Verification items for the finished model (mm, model axes). Round coordinates to 2 decimals unless told otherwise and drop trailing zeros. Write each loop counter-clockwise with the first axis right and the second up, starting at its lowest first coordinate (ties: lowest second). Pieces come first, ordered by that corner, then holes. Notation, with made-up numbers: M 22,-10 L 79,-10 A10 cw 79,7 Z; hole C 72,-22.75 d10. An arc over 180 degrees is marked long. One line per item, written item: value. Start each with the question number.
Item 1: Gauge pin test, flat end, axial feed: pin 1 (13 mm diameter, centred on x = -20.95, y = 10, fed in from +Z). Record the tip position at first contact, or that the pin passes through.
Item 2: Section check B-B, the plane x = -20.95. Record the cut outline in (y, z).
Item 3: Section check C-C, the plane z = 1.35. Record the cut outline in (x, y).
Item 4: Section check D-D, the plane x = 17. Record the cut outline in (y, z), then the cut area to 3 significant figures.
Item 5: Thickness scan on probe 1 along Y at (x, z) = (20.95, 1.3); probe 2 along X at (y, z) = (14, 4); probe 3 along Y at (x, z) = (-20.5, 1.6). Record the ranges inside material, lowest first. Write a range as from..to.
Item 6: Section check A-A, the plane y = 10. Record the cut outline in (x, z).
from build123d import *

# Parameters (mm, degrees)
SKETCH1_W           = 230
SKETCH1_H           = 90
BOSS_EXTRUDE1_DEPTH = 5
FILLET1_R           = 20
CUT_EXTRUDE1_REACH  = 125.592
SKETCH2_R           = 11
SKETCH2_R_2         = 16.75
CUT_EXTRUDE2_REACH  = 125.592
SKETCH3_R           = 4.65
SKETCH3_R_2         = 4.8


with BuildPart() as part:
    # Sketch1 → Boss-Extrude1 (new body)
    with BuildSketch(Plane.XY):
        Rectangle(SKETCH1_W, SKETCH1_H)
    extrude(amount=BOSS_EXTRUDE1_DEPTH)

    # Fillet1
    fillet1_edges = [part.edges().sort_by_distance(p)[0] for p in [
        (-115, 45, 2.5),
        (115, 45, 2.5),
    ]]
    fillet(fillet1_edges, radius=FILLET1_R)

    # Sketch2 → Cut-Extrude1 (cut, up to next)
    with BuildSketch(Plane.XY.offset(5), mode=Mode.PRIVATE) as cut_extrude1_sk1:
        with Locations((-20.95, 10)):
            Circle(SKETCH2_R)
    cut_extrude1_tool1 = extrude(cut_extrude1_sk1.sketch, amount=-CUT_EXTRUDE1_REACH, mode=Mode.PRIVATE) & part.part
    # Sketch2 → Cut-Extrude1 (cut, up to next)
    with BuildSketch(Plane.XY.offset(5), mode=Mode.PRIVATE) as cut_extrude1_sk2:
        with Locations((20.95, 10)):
            Circle(SKETCH2_R)
    cut_extrude1_tool2 = extrude(cut_extrude1_sk2.sketch, amount=-CUT_EXTRUDE1_REACH, mode=Mode.PRIVATE) & part.part
    # Sketch2 → Cut-Extrude1 (cut, up to next)
    with BuildSketch(Plane.XY.offset(5), mode=Mode.PRIVATE) as cut_extrude1_sk3:
        with Locations((49.976927154, -10)):
            Circle(SKETCH2_R_2)
    cut_extrude1_tool3 = extrude(cut_extrude1_sk3.sketch, amount=-CUT_EXTRUDE1_REACH, mode=Mode.PRIVATE) & part.part
    add(cut_extrude1_tool1.solids().sort_by_distance((-20.95, 10, 5))[0], mode=Mode.SUBTRACT)
    add(cut_extrude1_tool2.solids().sort_by_distance((20.95, 10, 5))[0], mode=Mode.SUBTRACT)
    add(cut_extrude1_tool3.solids().sort_by_distance((49.976927, -10, 5))[0], mode=Mode.SUBTRACT)

    # Sketch3 → Cut-Extrude2 (cut, up to next)
    with BuildSketch(Plane(origin=(0, 0, 0), x_dir=(-1, 0, 0), z_dir=(0, 0, -1)), mode=Mode.PRIVATE) as cut_extrude2_sk1:
        with Locations((-42.861480484, 27.315297382)):
            Circle(SKETCH3_R)
    cut_extrude2_tool1 = extrude(cut_extrude2_sk1.sketch, amount=-CUT_EXTRUDE2_REACH, mode=Mode.PRIVATE) & part.part
    # Sketch3 → Cut-Extrude2 (cut, up to next)
    with BuildSketch(Plane(origin=(0, 0, 0), x_dir=(-1, 0, 0), z_dir=(0, 0, -1)), mode=Mode.PRIVATE) as cut_extrude2_sk2:
        with Locations((-88.015918911, -8.560303387)):
            Circle(SKETCH3_R)
    cut_extrude2_tool2 = extrude(cut_extrude2_sk2.sketch, amount=-CUT_EXTRUDE2_REACH, mode=Mode.PRIVATE) & part.part
    # Sketch3 → Cut-Extrude2 (cut, up to next)
    with BuildSketch(Plane(origin=(0, 0, 0), x_dir=(-1, 0, 0), z_dir=(0, 0, -1)), mode=Mode.PRIVATE) as cut_extrude2_sk3:
        with Locations((-16.935196723, -27.604446885)):
            Circle(SKETCH3_R_2)
    cut_extrude2_tool3 = extrude(cut_extrude2_sk3.sketch, amount=-CUT_EXTRUDE2_REACH, mode=Mode.PRIVATE) & part.part
    add(cut_extrude2_tool1.solids().sort_by_distance((42.86148, 27.315297, 0))[0], mode=Mode.SUBTRACT)
    add(cut_extrude2_tool2.solids().sort_by_distance((88.015919, -8.560303, 0))[0], mode=Mode.SUBTRACT)
    add(cut_extrude2_tool3.solids().sort_by_distance((16.935197, -27.604447, 0))[0], mode=Mode.SUBTRACT)


solid = part.part
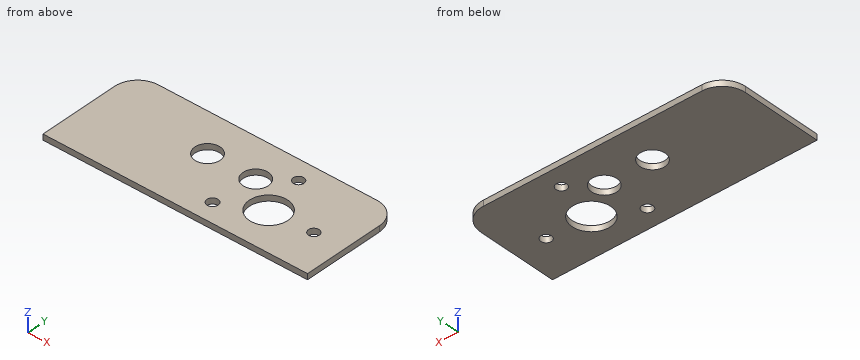
Response values:
1. pin 1: passes through
2. outline: M -45,0 L -1,0 L -1,5 L -45,5 Z; M 21,0 L 45,0 L 45,5 L 21,5 Z
3. outline: M -115,-45 L 115,-45 L 115,25 A20 ccw 95,45 L -95,45 A20 ccw -115,25 Z; hole C -20.95,10 d22; hole C 20.95,10 d22; hole C 16.94,-27.6 d9.6; hole C 49.98,-10 d33.5; hole C 42.86,27.32 d9.3; hole C 88.02,-8.56 d9.3
4. outline: M -45,0 L -32.4,0 L -32.4,5 L -45,5 Z; M -22.8,0 L -0.27,0 L -0.27,5 L -22.8,5 Z; M 20.27,0 L 45,0 L 45,5 L 20.27,5 Z
4. area: 299 mm2
5. probe 1: y = -45..-30.24, -24.97..-1, 21..45
5. probe 2: x = -115..-31.2, -10.7..10.7, 31.2..115
5. probe 3: y = -45..-0.99, 20.99..45
6. outline: M -115,0 L -31.95,0 L -31.95,5 L -115,5 Z; M -9.95,0 L 9.95,0 L 9.95,5 L -9.95,5 Z; M 31.95,0 L 115,0 L 115,5 L 31.95,5 Z
